```python
from build123d import *

# Parameters (mm, degrees)
SKETCH1_R           = 4.7625
BOSS_EXTRUDE1_DEPTH = 20
CUT_EXTRUDE1_DEPTH  = 7
SKETCH3_R           = 1.5875
CUT_EXTRUDE2_DEPTH  = 11


with BuildPart() as part:
    # Sketch1 → Boss-Extrude1 (new body)
    with BuildSketch(Plane(origin=(0, 0, 0), x_dir=(1, 0, 0), z_dir=(0, 1, 0))):
        Circle(SKETCH1_R)
    extrude(amount=BOSS_EXTRUDE1_DEPTH)

    # Sketch2 → Cut-Extrude1 (cut)
    with BuildSketch(Plane(origin=(0, 20, 0), x_dir=(1, 0, 0), z_dir=(0, 1, 0))):
        with BuildLine():
            Line((1.5, 2), (1.5, -2))
            ThreePointArc((1.5, -2), (-2.5, 0), (1.5, 2))
        make_face()
    extrude(amount=-CUT_EXTRUDE1_DEPTH, mode=Mode.SUBTRACT)

    # Sketch3 → Cut-Extrude2 (cut)
    with BuildSketch(Plane.XZ):
        Circle(SKETCH3_R)
    extrude(amount=-CUT_EXTRUDE2_DEPTH, mode=Mode.SUBTRACT)


solid = part.part
```
Build history of the part. All positions in model axes, mm. A direction names the side the tool comes from. Give positions to 0.01 mm unless a question says otherwise; leave off trailing zeros. Loops run counter-clockwise (first coordinate to the right, second up) from the corner with the lowest first, then second, coordinate; pieces in that order, holes last.
Item 1: Drill centre lines: line 1 (Z direction, x = 0, y = 15.25); line 2 (Z direction, x = 0, y = 5.5); line 3 (Y direction, x = -0.5, z = 0.25). Where is each one in solid material? Low to high.
Answers follow:
line 1: z = -4.76 to -2.5, 2.5 to 4.76
line 2: z = -4.76 to -1.59, 1.59 to 4.76
line 3: y = 11 to 13
Item 2: Slice it at A-A, the plane z = 0. List the corners of the cut face in (x, y).
Answers follow:
outline: (-4.76, 0) - (-1.59, 0) - (-1.59, 11) - (1.59, 11) - (1.59, 0) - (4.76, 0) - (4.76, 20) - (1.5, 20) - (1.5, 13) - (-2.5, 13) - (-2.5, 20) - (-4.76, 20) - close
Item 3: Slice it at C-C, the plane x = 0. List the corners of the cut face in (y, z), and give its area (3 significant figures).
Answers follow:
outline: (0, -4.76) - (20, -4.76) - (20, -2.5) - (13, -2.5) - (13, 2.5) - (20, 2.5) - (20, 4.76) - (0, 4.76) - (0, 1.59) - (11, 1.59) - (11, -1.59) - (0, -1.59) - close
area: 121 mm2
Item 4: Pull direction Z, two halves, no side cores. Call faces 4 (the face through (2, 20, 0)), 5 (the face through (1.5, 17, 0)), 6 (the face through (-3.78, 9.86, 2.9)): released by +Z, released by -Z, zero draft, split by the parting line, or undercut.
Answers follow:
face 4: zero draft
face 5: undercut
face 6: split by the parting line
Item 5: Flat gauge pins, fed straight in: pin 1 (3 mm diameter, centred on y = 10, z = -3.5, fed in from -X); pin 2 (1 mm diameter, centred on x = 0.5, z = 0, fed in from -Y); pin 3 (3 mm diameter, centred on x = -3, y = 5, fed in from -Z). Where does each tip first touch, or does it go through?
Answers follow:
pin 1: stops at x = -4.32
pin 2: stops at y = 11
pin 3: stops at z = -4.52
Item 6: Slice it at D-D, the plane y = 3.25. List the corners of the cut face in (x, z) (1 decimal).
Answers follow:
outline: circle Ø9.5 at (0, 0); hole circle Ø3.2 at (0, 0)
Item 7: Which spindle directions (+Z, -Z, +X, -X, +Y, -Y) get a long thin tool onto all of the face, cutting with end or side? Do faces 1 (the face through (0, 13, 0)), 2 (the face through (0, 11, 0)), 3 (the face through (2, 0, 0)). Say none if no direction does.
Answers follow:
face 1: +Y
face 2: -Y
face 3: +Z, -Z, +X, -X, -Y
Item 8: Slice it at B-B, the plane y = 13.5. List the corners of the cut face in (x, z) (1 decimal), and give its area (3 significant figures).
Answers follow:
outline: circle Ø9.5 at (0, 0); hole (1.5, -2) - (1.5, 2) arc R2.5 ccw (long way) to start
area: 54.4 mm2
